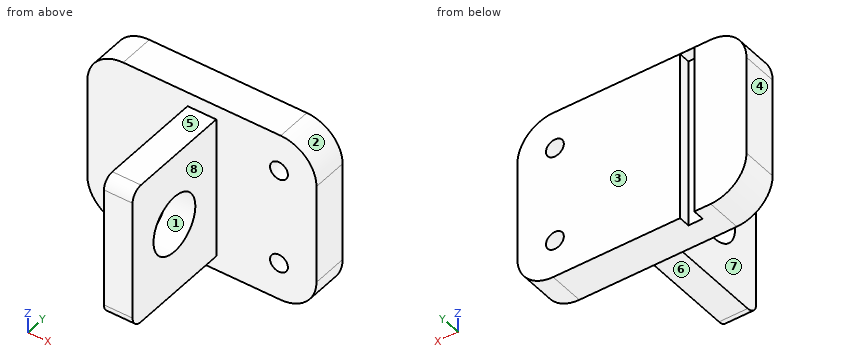
```python
from build123d import *

# Parameters (mm, degrees)
F0_W      = 101.6
F0_H      = 76.2
F1_DEPTH  = 15.875
F2_R      = 15.875
F3_R      = 3.9624
F4_DEPTH  = 25.4
F5_W      = 12.7
F5_H      = 63.5
F6_DEPTH  = 50.8
F7_R      = 5.08
F8_R      = 12.7
F9_DEPTH  = 25.4
F10_W     = 6.35
F10_H     = 76.149869
F11_DEPTH = 5.08


with BuildPart() as f1:
    # F0 (on Front) → F1 (new body)
    with BuildSketch(Plane.XZ):
        Rectangle(F0_W, F0_H)
    extrude(amount=F1_DEPTH)

    # F2
    f2_edges = [f1.edges().sort_by_distance(p)[0] for p in [
        (-50.8, -7.9375, 38.1),
        (50.8, -7.9375, 38.1),
        (50.8, -7.9375, -38.1),
        (-50.8, -7.9375, -38.1),
    ]]
    fillet(f2_edges, radius=F2_R)

    # F3 (on face) → F4 (cut)
    with BuildSketch(Plane.XZ.offset(15.875)):
        with Locations((34.163, -21.463)):
            Circle(F3_R)
        with Locations((34.163, 21.463)):
            Circle(F3_R)
    extrude(amount=-F4_DEPTH, mode=Mode.SUBTRACT)

    # F5 (on face) → F6 (join)
    with BuildSketch(Plane.XZ.offset(15.875)):
        Rectangle(F5_W, F5_H)
    extrude(amount=F6_DEPTH)

    # F7
    f7_edges = [f1.edges().sort_by_distance(p)[0] for p in [
        (0, -66.675, -31.75),
        (0, -66.675, 31.75),
    ]]
    fillet(f7_edges, radius=F7_R)

    # F8 (on face) → F9 (cut)
    with BuildSketch(Plane.YZ.offset(6.35)):
        with Locations((-41.275, 0)):
            Circle(F8_R)
    extrude(amount=-F9_DEPTH, mode=Mode.SUBTRACT)

    # F10 (on face) → F11 (cut)
    with BuildSketch(Plane.XZ):
        with Locations((-24.497632, -0.025066)):
            Rectangle(F10_W, F10_H)
    extrude(amount=F11_DEPTH, mode=Mode.SUBTRACT)


solid = f1.part
```
Check sheet for the modelled part. Datum: model origin and axes. Units: mm. Face numbers are marked on the shaded views. A direction names the side the tool comes from. Give positions to 0.01 mm unless a question says otherwise; leave off trailing zeros. Write each loop counter-clockwise with the first axis right and the second up, starting at its lowest first coordinate (ties: lowest second). Pieces come first, ordered by that corner, then holes. Notation, with made-up numbers: (72.25, 57) -> (89.25, 57) arc R30 cw to (89.25, 84) -> close; hole circle Ø7 at (55, 22.25). An arc over 180 degrees is marked (long way). Use CSV: the item, a comma, the result in double quotes. Start each with the question number.
Q1. Cross-section at C-C on z = -16. Enter the section's corners in (x, y) (3 decimals), and give its area (3 significant figures).
Q2. Cross-section at D-D on y = -10. Enter the section's corners in (x, z) (3 decimals).
Q3. Scan lines: line 1 along Y through (x, z) = (31, 33) (3 decimals); line 2 along X through (y, z) = (-18.5, 11.5); line 3 along X through (y, z) = (-12.5, 24). Record each from-to range of solid material in increasing order.
Q4. Cross-section at B-B on y = -36.5. Enter the section's corners in (x, z).
Q5. Tool access check on the marked faces 4, 5, 6, 7 and 8. Record the directions out of +Z, -Z, +X, -X, +Y, -Y that give a thin tool (end or side, any length) a straight path to the whole face; none if there is none.
Q6. Depth check by flat-ended pin: P1, Ø14, axis at x = -1, y = -32.5, coming from the -Z side; P2, Ø2.5, axis at x = -24.5, y = -2, coming from the -Z side; P3, Ø10, axis at x = -0.5, y = -37.5, coming from the +Z side. Enter the tip coordinate at first touch or a pass-through.
Q7. Cross-section at A-A on z = 0. Enter the section's corners in (x, y) (3 decimals).
Q8. Release check for a two-part mould opening along Y. For the marked faces 1, 2 and 3 record: +Y half, -Y half, draft (parallel to the pull), parting line (faces both ways), or undercut.
Working result:
1,outline,"(-50.8, -15.875) -> (-6.35, -15.875) -> (-6.35, -66.675) -> (6.35, -66.675) -> (6.35, -15.875) -> (50.8, -15.875) -> (50.8, 0) -> (-21.323, 0) -> (-21.323, -5.08) -> (-27.673, -5.08) -> (-27.673, 0) -> (-50.8, 0) -> close"
1,area,"2,230 mm^2"
2,outline,"(-50.8, -22.225) arc R15.875 ccw to (-34.925, -38.1) -> (34.925, -38.1) arc R15.875 ccw to (50.8, -22.225) -> (50.8, 22.225) arc R15.875 ccw to (34.925, 38.1) -> (-34.925, 38.1) arc R15.875 ccw to (-50.8, 22.225) -> close; hole circle Ø7.925 at (34.163, -21.463); hole circle Ø7.925 at (34.163, 21.463)"
3,line 1,"y = -15.875 to 0"
3,line 2,"x = -6.35 to 6.35"
3,line 3,"x = -50.7 to 31.12, 37.21 to 50.7"
4,outline,"(-6.35, -31.75) -> (6.35, -31.75) -> (6.35, -11.77) -> (-6.35, -11.77) -> close; (-6.35, 11.77) -> (6.35, 11.77) -> (6.35, 31.75) -> (-6.35, 31.75) -> close"
5,face 4,"+Z, -Z, -X, +Y, -Y"
5,face 5,"+Z, +X, -X, -Y"
5,face 6,"-Z, +X, -X, -Y"
5,face 7,"+Z, -Z, -X, -Y"
5,face 8,"+Z, -Z, +X, -Y"
6,P1,"stops at z = -31.75"
6,P2,"stops at z = 38.05"
6,P3,"stops at z = 31.75"
7,outline,"(-50.8, -15.875) -> (-6.35, -15.875) -> (-6.35, -28.575) -> (6.35, -28.575) -> (6.35, -15.875) -> (50.8, -15.875) -> (50.8, 0) -> (-21.323, 0) -> (-21.323, -5.08) -> (-27.673, -5.08) -> (-27.673, 0) -> (-50.8, 0) -> close; (-6.35, -66.675) -> (6.35, -66.675) -> (6.35, -53.975) -> (-6.35, -53.975) -> close"
8,face 1,"undercut"
8,face 2,"draft"
8,face 3,"+Y half"
